Autodesk Inventor part; units mm, degrees
ref_plane "YZ Plane" through (0, 0, 0) normal (1, 0, 0) x (0, 1, 0)
ref_plane "XZ Plane" through (0, 0, 0) normal (0, 1, 0) x (-1, 0, 0)
ref_plane "XY Plane" through (0, 0, 0) normal (0, 0, 1) x (1, 0, 0)
sketch "Sketch1" plane through (0, 0, 0) normal (0, 1, 0) x (-1, 0, 0)
  line L0 (-3.65, -50) -> (3.65, -50)
  line L1 (10, -43.65) -> (10, 43.65)
  line L2 (3.65, 50) -> (-3.65, 50)
  line L3 (-10, 43.65) -> (-10, -43.65)
  line L4 (-10, -50) -> (10, 50) construction
  line L5 (10, -50) -> (-10, 50) construction
  line L6 (37.1563, 0) -> (-27.0395, 0)
  circle A0 centre (0, 40) radius 5.25
  line L7 (0, 56.6322) -> (0, -75.9879)
  circle A1 centre (0, -40) radius 5.25
  arc A2 (10, 43.65) -> (3.65, 50) centre (3.65, 43.65) ccw
  arc A3 (-3.65, 50) -> (-10, 43.65) centre (-3.65, 43.65) ccw
  arc A4 (-10, -43.65) -> (-3.65, -50) centre (-3.65, -43.65) ccw
  arc A5 (3.65, -50) -> (10, -43.65) centre (3.65, -43.65) ccw
  circle A6 centre (0, 0) radius 2.54
  point P0 (0, 0)
  dimension "d0" = 100
  dimension "d1" = 20
  dimension "d2" = 10.5
  dimension "d3" = 80
  dimension "d4" = 6.35
  dimension "d7" = 5.08
extrude "Extrusion1" add sketch "Sketch1" along normal blind 6.35 contours A4 L3 L6 A6 L7 A1 L0 | L7 A1 A6 L6 L1 A5 L0 | L3 A3 L2 L7 A0 A6 L6 | L6 A6 L7 A0 L2 A2 L1
properties part number "Support_Plate"
Work out the finished part from the listing and answer in its coordinate system (mm). Coordinates: 2 decimals unless noted, no trailing zeros. Loops run counter-clockwise (first coordinate to the right, second up) from the corner with the lowest first, then second, coordinate; pieces in that order, holes last. Notation, with made-up numbers: (38.5, -23) - (78.5, -23) arc R16 cw to (78.5, 3) - close; hole circle Ø1 at (81, -20). An arc over 180 degrees is marked (long way). Use a Markdown table: item, result.
Item 1: Find section D-D, the plane z = 40. Determine the outline of the cut face in (x, y), and give its area (3 significant figures).
Evaluation:
| item | result |
|---|---|
| outline | (-10, 0) - (-5.25, 0) - (-5.25, 6.35) - (-10, 6.35) - close; (5.25, 0) - (10, 0) - (10, 6.35) - (5.25, 6.35) - close |
| area | 60.3 mm2 |
Item 2: Find section C-C, the plane y = 3.5. Determine the outline of the cut face in (x, z), and give its area (3 significant figures).
Evaluation:
| item | result |
|---|---|
| outline | (-10, -43.65) arc R6.35 ccw to (-3.65, -50) - (3.65, -50) arc R6.35 ccw to (10, -43.65) - (10, 43.65) arc R6.35 ccw to (3.65, 50) - (-3.65, 50) arc R6.35 ccw to (-10, 43.65) - close; hole circle Ø10.5 at (0, -40); hole circle Ø10.5 at (0, 40); hole circle Ø5.08 at (0, 0) |
| area | 1,770 mm2 |
Item 3: The mould has two halves that part along Z. Classify faces 1 (the flat face through (-4, 6.35, 1)), 2 (the cylindrical face through (0.33, 3.13, -2.52)), 3 (the flat face through (0, 3, 50)): +Z half, -Z half, draft (parallel to the pull), parting line (faces both ways), or undercut.
Evaluation:
| item | result |
|---|---|
| face 1 | draft |
| face 2 | undercut |
| face 3 | +Z half |
Item 4: Given pin 1 Ø9.5 at (x, z) = (0, -40) entering from -Y, flat-ended and moving along its own axis, determine where the tip first touches the part or whether it passes through.
Evaluation:
| item | result |
|---|---|
| pin 1 | passes through |
Item 5: Consider probe 1 along Z at (x, y) = (0, 2.5); probe 2 along X at (y, z) = (2.5, 40); probe 3 along Z at (x, y) = (3.5, 6.25). Determine where each line is inside the solid, lowest interval first. Write a range as from..to.
Evaluation:
| item | result |
|---|---|
| probe 1 | z = -50..-45.25, -34.75..-2.54, 2.54..34.75, 45.25..50 |
| probe 2 | x = -10..-5.25, 5.25..10 |
| probe 3 | z = -50..-43.91, -36.09..36.09, 43.91..50 |
Item 6: Find section B-B, the plane x = 0. Determine the outline of the cut face in (y, z).
Evaluation:
| item | result |
|---|---|
| outline | (0, -50) - (6.35, -50) - (6.35, -45.25) - (0, -45.25) - close; (0, -34.75) - (6.35, -34.75) - (6.35, -2.54) - (0, -2.54) - close; (0, 2.54) - (6.35, 2.54) - (6.35, 34.75) - (0, 34.75) - close; (0, 45.25) - (6.35, 45.25) - (6.35, 50) - (0, 50) - close |
Item 7: Find section A-A, the plane z = 0. Determine the outline of the cut face in (x, y).
Evaluation:
| item | result |
|---|---|
| outline | (-10, 0) - (-2.54, 0) - (-2.54, 6.35) - (-10, 6.35) - close; (2.54, 0) - (10, 0) - (10, 6.35) - (2.54, 6.35) - close |
